Part model, mm, in its own coordinate system. A direction names the side the tool comes from. Coordinates: 2 decimals unless noted, no trailing zeros. Order: outer loops, then holes, each group sorted by start corner. A loop starts at its lowest first (then second) coordinate and runs counter-clockwise, first axis right, second up.
1) Tool access for faces 4 (the flat face through (0, 10.5, 0)), 5 (the flat face through (-9, 4.5, -9)): list every direction of +Z, -Z, +X, -X, +Y, -Y with a clear straight run to the whole face (end or side of a thin tool).
2) Cut at B-B (x = 0). List the corners of the cut face in (y, z).
3) Cut at C-C (x = 8.5). List the corners of the cut face in (y, z), and give its area (3 significant figures).
4) Cut at A-A (z = 0). List the corners of the cut face in (x, y), and give its area (3 significant figures).
5) Cut at D-D (z = -4). List the corners of the cut face in (x, y).
6) Mould opens along X. For faces 1 (the cylindrical face through (-2.38, 7.46, -10.74)), 2 (the cylindrical face through (8.14, 1.726, 15.867)), 3 (the flat face through (0, 0, 0)) say: +X half, -X half, draft (parallel to the pull), parting line (faces both ways), or undercut.
7) Wall check: L1, parallel to Z at x = 8.5, y = 1.4; L2, parallel to Z at x = 9, y = 0.75; L3, parallel to Y at x = 13.5, z = 3.5. Give the ranges that are in metal, low to high.
8) Pin check, flat tips, straight feed: pin 1 Ø4 at (x, y) = (-8, 5.5) entering from -Z; pin 2 Ø1.5 at (x, y) = (-1, 6) entering from +Z; pin 3 Ø1 at (x, y) = (4, 3.5) entering from +Z; pin 4 Ø12 at (x, z) = (-9.5, 6) entering from +Y. Stop position of each tip, or through.
Autodesk Inventor part; units mm, degrees
ref_plane "YZ Plane" through (0, 0, 0) normal (1, 0, 0) x (0, 1, 0)
ref_plane "XZ Plane" through (0, 0, 0) normal (0, 1, 0) x (-1, 0, 0)
ref_plane "XY Plane" through (0, 0, 0) normal (0, 0, 1) x (1, 0, 0)
sketch "Sketch1" plane through (0, 0, 0) normal (0, 1, 0) x (-1, 0, 0)
  circle A0 centre (0, 0) radius 20
  dimension "d0" = 40
extrude "Extrusion1" add sketch "Sketch1" along normal blind 4.5
sketch "Sketch2" plane through (0, 4.5, 0) normal (0, 1, 0) x (1, 0, 0)
  circle A0 centre (0, 0) radius 11
  dimension "d3" = 22
extrude "Extrusion2" add sketch "Sketch2" along normal blind 6
sketch "Sketch3" plane through (0, 4.5, 0) normal (0, 1, 0) x (1, 0, 0)
  line L0 (0, -21.0157) -> (0, 24.936) construction
  line L1 (-27.3573, 0) -> (21.7209, 0) construction
  circle A0 centre (0, 0) radius 17 construction
  point P0 (-17, 0)
  point P1 (8.5, -14.7224)
  point P2 (8.5, 14.7224)
  dimension "d6" = 34
  dimension "d9" = 360
hole "Hole1" at (-17, 4.5, 0) at (8.5, 4.5, 14.7224) at (8.5, 4.5, -14.7224) direction (0, -1, 0) diameter 2.4 end through all countersink diameter 4.4 countersink angle 90
properties part number "EChem _S200 Cap Base"
Geometry check:
1. face 4: +Z, -Z, +X, -X, +Y
1. face 5: +Y
2. outline: (0, -20) - (4.5, -20) - (4.5, -11) - (10.5, -11) - (10.5, 11) - (4.5, 11) - (4.5, 20) - (0, 20) - close
3. outline: (0, -18.1) - (4.5, -18.1) - (4.5, -16.92) - (3.5, -15.92) - (0, -15.92) - close; (0, -13.52) - (3.5, -13.52) - (4.5, -12.52) - (4.5, -6.98) - (10.5, -6.98) - (10.5, 6.98) - (4.5, 6.98) - (4.5, 12.52) - (3.5, 13.52) - (0, 13.52) - close; (0, 15.92) - (3.5, 15.92) - (4.5, 16.92) - (4.5, 18.1) - (0, 18.1) - close
3. area: 223 mm2
4. outline: (-20, 0) - (-18.2, 0) - (-18.2, 3.5) - (-19.2, 4.5) - (-20, 4.5) - close; (-15.8, 0) - (20, 0) - (20, 4.5) - (11, 4.5) - (11, 10.5) - (-11, 10.5) - (-11, 4.5) - (-14.8, 4.5) - (-15.8, 3.5) - close
4. area: 300 mm2
5. outline: (-19.6, 0) - (19.6, 0) - (19.6, 4.5) - (10.25, 4.5) - (10.25, 10.5) - (-10.25, 10.5) - (-10.25, 4.5) - (-19.6, 4.5) - close
6. face 1: parting line
6. face 2: undercut
6. face 3: draft
7. L1: z = -18.1 to -15.92, -13.52 to 13.52, 15.92 to 18.1
7. L2: z = -17.86 to -15.81, -13.63 to 13.63, 15.81 to 17.86
7. L3: y = 0 to 4.5
8. pin 1: stops at z = -18.99
8. pin 2: stops at z = 11
8. pin 3: stops at z = 19.69
8. pin 4: stops at y = 10.5
